from build123d import *

# Parameters (mm, degrees)
SKETCH_1_R          = 5
SKETCH_1_R_2        = 2.75
EXTRUDE_1_DEPTH     = 10
SKETCH_2_R          = 2
CUT_EXTRUDE_1_DEPTH = 20
SKETCH_4_R          = 5
CUT_EXTRUDE_3_DEPTH = 5


with BuildPart() as part:
    # 스케치1 → 보스-돌출1 (new body)
    with BuildSketch(Plane.XY):
        with BuildLine():
            Line((25, 0), (25, 42))
            Line((25, 42), (-25, 42))
            Line((-25, 42), (-25, 0))
            ThreePointArc((-25, 0), (0, -25), (25, 0))
        make_face()
        Circle(SKETCH_1_R, mode=Mode.SUBTRACT)
        with Locations((0, -13.5)):
            Circle(SKETCH_1_R_2, mode=Mode.SUBTRACT)
        with Locations((-11.691342951, -6.75)):
            Circle(SKETCH_1_R_2, mode=Mode.SUBTRACT)
        with Locations((-11.691342951, 6.75)):
            Circle(SKETCH_1_R_2, mode=Mode.SUBTRACT)
        with Locations((0, 13.5)):
            Circle(SKETCH_1_R_2, mode=Mode.SUBTRACT)
        with Locations((11.691342951, 6.75)):
            Circle(SKETCH_1_R_2, mode=Mode.SUBTRACT)
        with Locations((11.691342951, -6.75)):
            Circle(SKETCH_1_R_2, mode=Mode.SUBTRACT)
    extrude(amount=EXTRUDE_1_DEPTH)

    # 스케치2 → 컷-돌출1 (cut)
    with BuildSketch(Plane(origin=(0, 42, 0), x_dir=(1, 0, 0), z_dir=(0, 1, 0))):
        with Locations(Location((0, -5, 0), (0, 0, 270))):
            Circle(SKETCH_2_R)
        with Locations(Location((15, -5, 0), (0, 0, 270))):
            Circle(SKETCH_2_R)
        with Locations(Location((-15, -5, 0), (0, 0, 270))):
            Circle(SKETCH_2_R)
    extrude(amount=-CUT_EXTRUDE_1_DEPTH, mode=Mode.SUBTRACT)

    # 스케치4 → 컷-돌출3 (cut)
    with BuildSketch(Plane.XY.offset(10)):
        with Locations((0, 13.5)):
            Circle(SKETCH_4_R)
        with Locations((11.691342951, 6.75)):
            Circle(SKETCH_4_R)
        with Locations((11.691342951, -6.75)):
            Circle(SKETCH_4_R)
        with Locations((0, -13.5)):
            Circle(SKETCH_4_R)
        with Locations((-11.691342951, -6.75)):
            Circle(SKETCH_4_R)
        with Locations((-11.691342951, 6.75)):
            Circle(SKETCH_4_R)
    extrude(amount=-CUT_EXTRUDE_3_DEPTH, mode=Mode.SUBTRACT)


solid = part.part
CAD build for the part. Positions are in the model's coordinates, mm. A direction names the side the tool comes from. Coordinates: 2 decimals unless noted, no trailing zeros. Write each loop counter-clockwise with the first axis right and the second up, starting at its lowest first coordinate (ties: lowest second). Pieces come first, ordered by that corner, then holes. Notation, with made-up numbers: M 27,69.5 L 64,69.5 A15 ccw 64,80.5 Z; hole C 8.25,26.25 d2. An arc over 180 degrees is marked long. Answer as a JSON object with one key per item and string values. Group by question number.
1) Pin check, flat tips, straight feed: pin 1 Ø2.5 at (x, z) = (0, 5) entering from -Y; pin 2 Ø8 at (x, y) = (0, 13.5) entering from +Z; pin 3 Ø1.2 at (x, z) = (-0.5, 4.5) entering from +Y. Stop position of each tip, or through.
2) Saw through at D-D (y = 13.5). Write the cut outline in (x, z).
3) Saw through at A-A (x = 0). Write the cut outline in (y, z), plus the area to 3 significant figures.
4) Saw through at B-B (y = 6.75). Write the cut outline in (x, z), plus the area to 3 significant figures.
5) Saw through at C-C (z = 8.75). Write the cut outline in (x, y).
6) Tool access for faces 1 (the face through (14, -9, 5)), 2 (the face through (-10.42, 4.31, 2.46)), 3 (the face through (0, 32, 3)): list every direction of +Z, -Z, +X, -X, +Y, -Y with a clear straight run to the whole face (end or side of a thin tool).
7) Wall check: line 1 (X direction, y = 31, z = 5); line 2 (Y direction, x = 1.5, z = 4.5); line 3 (Y direction, x = -9.5, z = 3.25). Give the ranges that are in metal, low to high. Write a range as from..to.
8) Mould opens along Z. For faces 4 (the face through (0.3, 42, 2.7)), 5 (the face through (0, 22, 5)), 6 (the face through (2, 11, 5)) say: +Z half, -Z half, draft (parallel to the pull), parting line (faces both ways), or undercut.
Values follow:
{
 "1": {"pin 1": "stops at y = -25", "pin 2": "stops at z = 5", "pin 3": "stops at y = 22"},
 "2": {"outline": "M -25,0 L -2.75,0 L -2.75,5 L -5,5 L -5,10 L -25,10 Z; M 2.75,0 L 25,0 L 25,10 L 5,10 L 5,5 L 2.75,5 Z"},
 "3": {"outline": "M -25,0 L -16.25,0 L -16.25,5 L -18.5,5 L -18.5,10 L -25,10 Z; M -10.75,0 L -5,0 L -5,10 L -8.5,10 L -8.5,5 L -10.75,5 Z; M 5,0 L 10.75,0 L 10.75,5 L 8.5,5 L 8.5,10 L 5,10 Z; M 16.25,0 L 42,0 L 42,3 L 22,3 L 22,7 L 42,7 L 42,10 L 18.5,10 L 18.5,5 L 16.25,5 Z", "area": "335 mm2"},
 "4": {"outline": "M -25,0 L -14.44,0 L -14.44,5 L -16.69,5 L -16.69,10 L -25,10 Z; M -8.94,0 L 8.94,0 L 8.94,5 L 6.69,5 L 6.69,10 L -6.69,10 L -6.69,5 L -8.94,5 Z; M 14.44,0 L 25,0 L 25,10 L 16.69,10 L 16.69,5 L 14.44,5 Z", "area": "345 mm2"},
 "5": {"outline": "M -25,0 A25 ccw 25,0 L 25,42 L -25,42 Z; hole C -11.69,-6.75 d10; hole C -11.69,6.75 d10; hole C 0,-13.5 d10; hole C 0,0 d10; hole C 0,13.5 d10; hole C 11.69,-6.75 d10; hole C 11.69,6.75 d10"},
 "6": {"face 1": "+Z", "face 2": "+Z, -Z", "face 3": "+Y"},
 "7": {"line 1": "x = -25..-17, -13..-2, 2..13, 17..25", "line 2": "y = -24.95..-15.8, -11.2..-4.77, 4.77..11.2, 15.8..22", "line 3": "y = -23.12..-8.41, -5.09..5.09, 8.41..42"},
 "8": {"face 4": "draft", "face 5": "undercut", "face 6": "+Z half"}
}
